```python
from build123d import *

# Parameters (mm, degrees)
SKETCH_SPINDLE_SKELETON_W      = 1.000000064
SKETCH_SPINDLE_SKELETON_H      = 10.1187
CUT_CENTER_DEPTH               = 53.414934066
CUT_CENTER_DEPTH_BACK          = 53.414934066
SKETCH_CENTER_CUT_R            = 12.5
CBORE_FOR_M6_SHCS1_D           = 6.6
CBORE_FOR_M6_SHCS1_CBORE_D     = 11
CBORE_FOR_M6_SHCS1_CBORE_DEPTH = 6
CIRPATTERN1_COUNT              = 6
SKETCH1_R                      = 14.25575
CUT_EXTRUDE1_DEPTH             = 3.9624
CUT_EXTRUDE2_DEPTH             = 6
CIRPATTERN2_COUNT              = 6


with BuildPart() as part:
    # Sketch Spindle Skeleton → Main Revolve (revolve)
    with BuildSketch(Plane(origin=(0, 0, 0), x_dir=(0, 0, -1), z_dir=(1, 0, 0)), mode=Mode.PRIVATE) as main_revolve_sk:
        Polygon((-25.304999936, 12.5), (-25.304999936, 9.525), (-16.304999902, 9.525), (-16.304999902, 36.5125), (-25.304999936, 36.5125), (-25.304999936, 22.6187), (-26.304999936, 22.6187), (-26.304999936, 12.5), align=None)
        with Locations((-26.804999968, 17.55935)):
            Rectangle(SKETCH_SPINDLE_SKELETON_W, SKETCH_SPINDLE_SKELETON_H)
    revolve(main_revolve_sk.sketch.rotate(Axis((0, 0, 1000), (0, 0, -1)), 90), axis=Axis((0, 0, 1000), (0, 0, -1)))

    # Sketch Center Cut → Cut Center (cut, two sides: drawn at the far end of the back side and taken through both)
    with BuildSketch(Plane.XY.offset(25.304999936).offset(-CUT_CENTER_DEPTH_BACK)):
        Circle(SKETCH_CENTER_CUT_R)
    extrude(amount=CUT_CENTER_DEPTH + CUT_CENTER_DEPTH_BACK, mode=Mode.SUBTRACT)

    # CBORE for M6 SHCS1 (through all)
    with Locations(Plane(origin=(0, 0, 16.304999902), x_dir=(-1, 0, 0), z_dir=(0, 0, -1))):
        with Locations((0, 30.565600032)):
            cbore_for_m6_shcs1 = CounterBoreHole(CBORE_FOR_M6_SHCS1_D / 2, CBORE_FOR_M6_SHCS1_CBORE_D / 2, CBORE_FOR_M6_SHCS1_CBORE_DEPTH)

    # CirPattern1: CBORE for M6 SHCS1 ×6 about axis
    cirpattern1_axis = Axis((0, 0, 0), (0, 0, 1))
    for i in range(1, CIRPATTERN1_COUNT):
        add(cbore_for_m6_shcs1.rotate(cirpattern1_axis, i * 360 / CIRPATTERN1_COUNT), mode=Mode.SUBTRACT)

    # Sketch1 → Cut-Extrude1 (cut)
    with BuildSketch(Plane(origin=(0, 0, 16.304999902), x_dir=(-1, 0, 0), z_dir=(0, 0, -1))):
        Circle(SKETCH1_R)
    extrude(amount=-CUT_EXTRUDE1_DEPTH, mode=Mode.SUBTRACT)

    # Sketch2 → Cut-Extrude2 (cut)
    with BuildSketch(Plane(origin=(0, 0, 16.304999902), x_dir=(-1, 0, 0), z_dir=(0, 0, -1))):
        with BuildLine():
            ThreePointArc((5.5, 30.565600032), (5.416442642, 29.610535055), (5.168309414, 28.684489244))
            Line((5.168309414, 28.684489244), (7.71724355, 35.687628224))
            ThreePointArc((7.71724355, 35.687628224), (3.88060116, 36.305696397), (0, 36.5125))
            Line((0, 36.5125), (0, 36.065600032))
            ThreePointArc((0, 36.065600032), (3.889087297, 34.454687329), (5.5, 30.565600032))
        make_face()
        with BuildLine():
            Line((-7.71724355, 35.687628224), (-5.168309414, 28.684489244))
            ThreePointArc((-5.168309414, 28.684489244), (-4.505336244, 33.720270432), (0, 36.065600032))
            Line((0, 36.065600032), (0, 36.5125))
            ThreePointArc((0, 36.5125), (-3.88060116, 36.305696397), (-7.71724355, 35.687628224))
        make_face()
    cut_extrude2 = extrude(amount=-CUT_EXTRUDE2_DEPTH, mode=Mode.SUBTRACT)

    # CirPattern2: Cut-Extrude2 ×6 about axis
    cirpattern2_axis = Axis((0, 0, 0), (0, 0, 1))
    for i in range(1, CIRPATTERN2_COUNT):
        add(cut_extrude2.rotate(cirpattern2_axis, i * 360 / CIRPATTERN2_COUNT), mode=Mode.SUBTRACT)


solid = part.part
```
Verification items for the finished model (mm, model axes). A direction names the side the tool comes from. Round coordinates to 2 decimals unless told otherwise and drop trailing zeros. Write each loop counter-clockwise with the first axis right and the second up, starting at its lowest first coordinate (ties: lowest second). Pieces come first, ordered by that corner, then holes.
1. Section check C-C on z = 18.5. Enter the section's corners in (x, y) (1 decimal).
2. Scan lines: L1, parallel to Y at x = 0, z = 23.6; L2, parallel to Y at x = -22.5, z = 18.5; L3, parallel to Y at x = 23.5, z = 18.75. Record each from-to range of solid material in increasing order.
3. Draft check along Y on faces 1 (the flat face through (31.147, 10.522, 19.263)), 2 (the cylindrical face through (-21.755, -12.452, 19.263)), 3 (the flat face through (-31.147, -10.522, 19.263)). Enter one of: +Y half, -Y half, draft (parallel to the pull), parting line (faces both ways), or undercut.
4. Section check D-D on z = 23.25. Enter the section's corners in (x, y) (1 decimal).
5. Access from +Z, -Z, +X, -X, +Y, -Y to the whole of each face (thin tool, end or side, straight path). Record for faces 4 (the flat face through (24.686, -21.713, 19.263)), 5 (the flat face through (-6.425, 32.137, 19.263)), 6 (the flat face through (-17, 16, 25.305)), 7 (the flat face through (-24.686, 21.713, 19.263)), 8 (the flat face through (0, -13, 20.267)).
6. Section check B-B on x = 0. Enter the section's corners in (y, z) (1 decimal), plus the area to 3 significant figures.
7. Section check A-A on y = 0. Enter the section's corners in (x, z) (1 decimal).
8. Gauge pin test, flat ends, axial feed: P1, Ø4, axis at x = -29, y = -20.5, coming from the -Z side (3 decimals); P2, Ø2, axis at y = -4.5, z = 24.5, coming from the -X side; P3, Ø1.5, axis at y = 8.5, z = 17.5, coming from the -X side. Record the tip position at first contact, or that the pin passes through.
Answer:
1. outline: (-34.8, -11.2) - (-27.4, -9.9) arc R5.5 cw to (-22.3, -18.8) - (-27, -24.5) arc R36.5 ccw to (-7.7, -35.7) - (-5.2, -28.7) arc R5.5 cw to (5.2, -28.7) - (7.7, -35.7) arc R36.5 ccw to (27, -24.5) - (22.3, -18.8) arc R5.5 cw to (27.4, -9.9) - (34.8, -11.2) arc R36.5 ccw to (34.8, 11.2) - (27.4, 9.9) arc R5.5 cw to (22.3, 18.8) - (27, 24.5) arc R36.5 ccw to (7.7, 35.7) - (5.2, 28.7) arc R5.5 cw to (-5.2, 28.7) - (-7.7, 35.7) arc R36.5 ccw to (-27, 24.5) - (-22.3, 18.8) arc R5.5 cw to (-27.4, 9.9) - (-34.8, 11.2) arc R36.5 ccw to start; hole circle Ø28.5 at (0, 0)
2. L1: y = -36.51 to -33.87, -27.27 to -12.5, 12.5 to 27.27, 33.87 to 36.51
2. L2: y = -28.76 to -19.11, -11.48 to 11.48, 19.11 to 28.76
2. L3: y = -27.94 to -20.3, -10.65 to 10.65, 20.3 to 27.94
3. face 1: +Y half
3. face 2: undercut
3. face 3: -Y half
4. outline: circle Ø73 at (0, 0); hole circle Ø6.6 at (-26.5, -15.3); hole circle Ø6.6 at (-26.5, 15.3); hole circle Ø25 at (0, 0); hole circle Ø6.6 at (0, -30.6); hole circle Ø6.6 at (0, 30.6); hole circle Ø6.6 at (26.5, -15.3); hole circle Ø6.6 at (26.5, 15.3)
5. face 4: -Z, +X
5. face 5: -Z, +Y
5. face 6: +Z
5. face 7: -Z, -X
5. face 8: -Z
6. outline: (-36.5, 22.3) - (-33.9, 22.3) - (-33.9, 25.3) - (-36.5, 25.3) - close; (-27.3, 22.3) - (-25.1, 22.3) - (-25.1, 16.3) - (-14.3, 16.3) - (-14.3, 20.3) - (-12.5, 20.3) - (-12.5, 27.3) - (-22.6, 27.3) - (-22.6, 25.3) - (-27.3, 25.3) - close; (12.5, 20.3) - (14.3, 20.3) - (14.3, 16.3) - (25.1, 16.3) - (25.1, 22.3) - (27.3, 22.3) - (27.3, 25.3) - (22.6, 25.3) - (22.6, 27.3) - (12.5, 27.3) - close; (33.9, 22.3) - (36.5, 22.3) - (36.5, 25.3) - (33.9, 25.3) - close
6. area: 282 mm2
7. outline: (-36.5, 16.3) - (-14.3, 16.3) - (-14.3, 20.3) - (-12.5, 20.3) - (-12.5, 27.3) - (-22.6, 27.3) - (-22.6, 25.3) - (-36.5, 25.3) - close; (12.5, 20.3) - (14.3, 20.3) - (14.3, 16.3) - (36.5, 16.3) - (36.5, 25.3) - (22.6, 25.3) - (22.6, 27.3) - (12.5, 27.3) - close
8. P1: stops at z = 22.305
8. P2: stops at x = -36.34
8. P3: stops at x = -35.68
